from build123d import *

# Parameters (mm, degrees)
F2_DEPTH  = 22.7
F3_W      = 4.7
F3_H      = 4.3
F3_H_2    = 15.9
F4_DEPTH  = 11.801
F6_R      = 2.3
F7_DEPTH  = 4
F8_DEPTH  = 7.2
F9_R      = 1.25
F10_DEPTH = 5


with BuildPart() as f2:
    # F1 (on face) → F2 (new body)
    with BuildSketch(Plane.XY):
        with BuildLine():
            ThreePointArc((1.540066, 6.55), (3.3, 5.9), (1.540066, 5.25))
            Line((1.540066, 5.25), (0, 5.25))
            Line((0, 5.25), (0, 0))
            Line((0, 0), (15.95, 0))
            Line((15.95, 0), (15.95, 11.8))
            Line((15.95, 11.8), (0, 11.8))
            Line((0, 11.8), (0, 6.55))
            Line((0, 6.55), (1.540066, 6.55))
        make_face()
    extrude(amount=F2_DEPTH)

    # F3 (on face) → F4 (cut, through all)
    with BuildSketch(Plane(origin=(0, 11.8, 0), x_dir=(-1, 0, 0), z_dir=(0, 1, 0))):
        with Locations((-2.35, 2.15)):
            Rectangle(F3_W, F3_H)
        with Locations((-2.35, 14.75)):
            Rectangle(F3_W, F3_H_2)
    extrude(amount=-F4_DEPTH, mode=Mode.SUBTRACT)

    # F5: F2 across face


with BuildPart() as f2_1:
    add(f2.part)
    add(f2.part.mirror(Plane(origin=(15.95, 5.9, 11.35), x_dir=(0, 1, 0), z_dir=(1, 0, 0))))

    # F6 (on face) → F7 (join)
    with BuildSketch(Plane(origin=(0, 0, 0), x_dir=(1, 0, 0), z_dir=(0, 0, -1))):
        with BuildLine():
            Line((16.899756, -3.455402), (15.969724, -3.455402))
            ThreePointArc((15.969724, -3.455402), (13.792716, -0.938492), (10.6, 0))
            ThreePointArc((10.6, 0), (6.42807, -1.72807), (4.7, -5.9))
            ThreePointArc((4.7, -5.9), (6.42807, -10.07193), (10.6, -11.8))
            ThreePointArc((10.6, -11.8), (13.741109, -10.89434), (15.917887, -8.455402))
            Line((15.917887, -8.455402), (16.899756, -8.455402))
            ThreePointArc((16.899756, -8.455402), (19.399756, -5.955402), (16.899756, -3.455402))
        make_face()
        with Locations((10.6, -5.9)):
            Circle(F6_R, mode=Mode.SUBTRACT)
    extrude(amount=F7_DEPTH)

    # F6 (on face) → F8 (join)
    with BuildSketch(Plane(origin=(0, 0, 0), x_dir=(1, 0, 0), z_dir=(0, 0, -1))):
        with Locations((10.6, -5.9)):
            Circle(F6_R)
    extrude(amount=F8_DEPTH)

    # F9 (on face) → F10 (cut)
    with BuildSketch(Plane(origin=(0, 0, -7.2), x_dir=(1, 0, 0), z_dir=(0, 0, -1))):
        with Locations((10.6, -5.9)):
            Circle(F9_R)
    extrude(amount=-F10_DEPTH, mode=Mode.SUBTRACT)


solid = f2_1.part
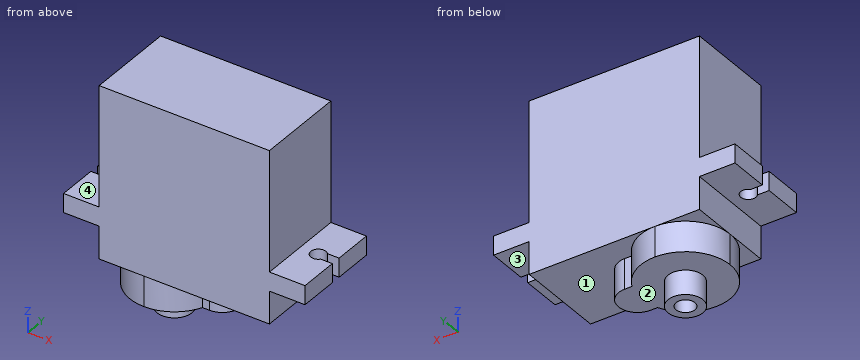
Check sheet for the modelled part. Datum: model origin and axes. Units: mm. Face numbers are marked on the shaded views. A direction names the side the tool comes from. Round coordinates to 2 decimals unless told otherwise and drop trailing zeros. Order: outer loops, then holes, each group sorted by start corner. A loop starts at its lowest first (then second) coordinate and runs counter-clockwise, first axis right, second up.
Q1. Set-up check for the marked faces 1, 2, 3 and 4: record each of +Z, -Z, +X, -X, +Y, -Y from which the full face is reachable in a straight line by a thin tool's end or side.
Filled sheet:
face 1: -Z, +X
face 2: -Z
face 3: -Z, +X, +Y, -Y
face 4: +Z, -X, +Y, -Y
Q2. Cross-section at D-D, the plane y = 0.5. Enter the section's corners in (x, z), plus the area to 3 significant figures.
Filled sheet:
outline: (0, 4.3) - (4.7, 4.3) - (4.7, 0) - (8.22, 0) - (8.22, -4) - (12.98, -4) - (12.98, 0) - (27.2, 0) - (27.2, 4.3) - (31.9, 4.3) - (31.9, 6.8) - (27.2, 6.8) - (27.2, 22.7) - (4.7, 22.7) - (4.7, 6.8) - (0, 6.8) - close
area: 553 mm2
Q3. Cross-section at C-C, the plane x = 18. Enter the section's corners in (y, z), plus the area to 3 significant figures.
Filled sheet:
outline: (0, 0) - (3.71, 0) - (3.71, -4) - (8.2, -4) - (8.2, 0) - (11.8, 0) - (11.8, 22.7) - (0, 22.7) - close
area: 286 mm2
Q4. Cross-section at B-B, the plane z = -3. Enter the section's corners in (x, y), plus the area to 3 significant figures.
Filled sheet:
outline: (10.6, 11.8) arc R5.9 ccw (long way) to (15.97, 3.46) - (16.9, 3.46) arc R2.5 ccw to (16.9, 8.46) - (15.92, 8.46) arc R5.9 ccw to start; hole circle Ø2.5 at (10.6, 5.9)
area: 117 mm2
Q5. Depth check by flat-ended pin: P1, Ø1.5, axis at x = 6.5, z = -0.5, coming from the +Y side; P2, Ø0.8, axis at x = 16.5, z = -1, coming from the +Y side; P3, Ø4, axis at x = 3.5, y = 7, coming from the -Z side; P4, Ø0.8, axis at x = 10.5, y = 5.5, coming from the -Z side. Enter the tip coordinate at first touch or a pass-through.
Filled sheet:
P1: stops at y = 11.8
P2: stops at y = 8.46
P3: stops at z = -4
P4: stops at z = -2.2
Q6. Scan lines: L1, parallel to Y at x = 10.6, z = -5.2; L2, parallel to X at y = 5.9, z = -4.85; L3, parallel to Y at x = 2.3, z = 5.7. Record each from-to range of solid material in increasing order.
Filled sheet:
L1: y = 3.6 to 4.65, 7.15 to 8.2
L2: x = 8.3 to 9.35, 11.85 to 12.9
L3: y = 0 to 4.9, 6.9 to 11.8
Q7. Cross-section at A-A, the plane x = 29.6. Enter the section's corners in (y, z).
Filled sheet:
outline: (0, 4.3) - (4.9, 4.3) - (4.9, 6.8) - (0, 6.8) - close; (6.9, 4.3) - (11.8, 4.3) - (11.8, 6.8) - (6.9, 6.8) - close
